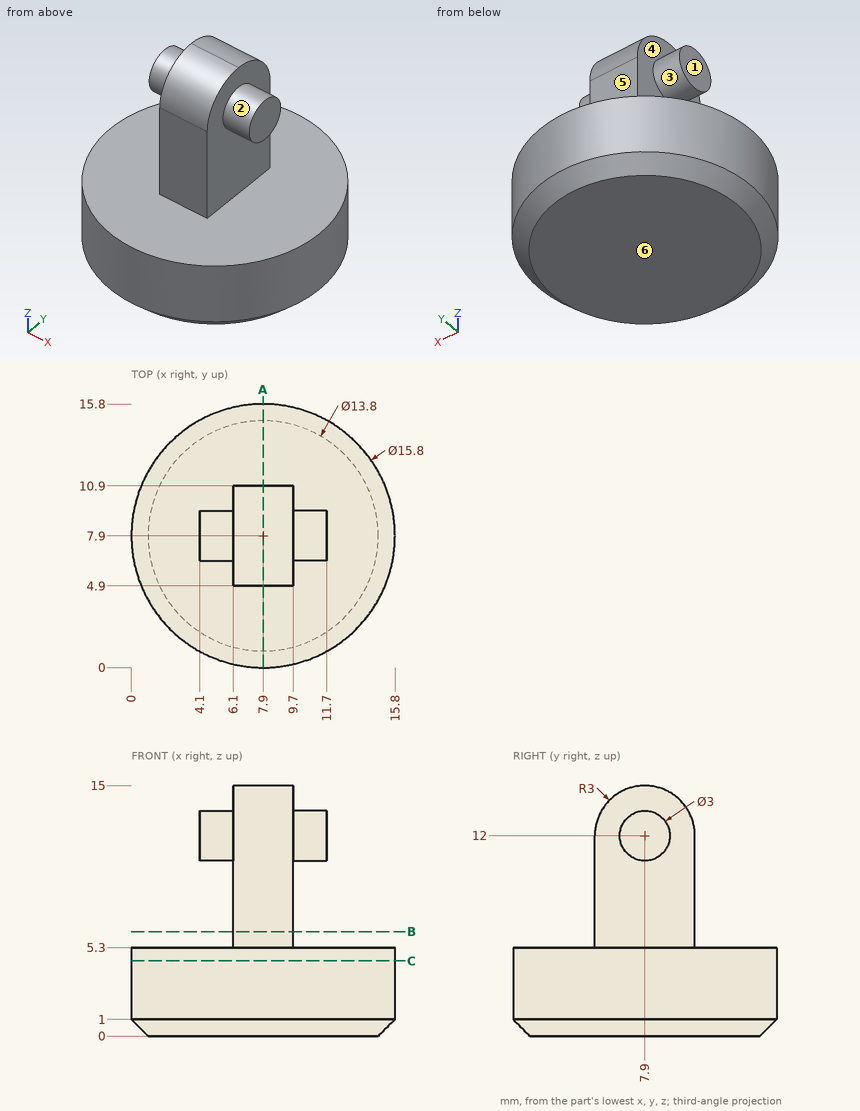
Drawing for the job (mm, zero at the part's lowest x, y, z). A direction names the side the tool comes from. Give positions to 0.01 mm unless a question says otherwise; leave off trailing zeros. Write each loop counter-clockwise with the first axis right and the second up, starting at its lowest first coordinate (ties: lowest second). Pieces come first, ordered by that corner, then holes. Notation, with made-up numbers: M 58,31 L 64,31 A18 ccw 64,57 Z; hole C 89.5,-39 d2. An arc over 180 degrees is marked long. Return JSON: item names as keys, results as strings. Group by question number.
(1) Band-saw the part on C-C (z = 4.5). Give the cut face in (x, y).
(2) Band-saw the part on B-B (z = 6.25). Give the cut face in (x, y).
(3) Mould opens along Z. For the marked faces 4, 5 and 6 say: pulls with the +Z half, pulls with the -Z half, needs draft (parallel to the pull), parting line crosses it, or undercut.
(4) Drill centre lines: L1, parallel to X at y = 5.5, z = 11.5; L2, parallel to Z at x = 5.25, y = 14; L3, parallel to Z at x = 11, y = 8. Where is each one in solid material? Low to high. Write a range as [from, to].
(5) Flat gauge pins, fed straight in: pin 1 Ø1.1 at (x, z) = (7.5, 9) entering from -Y; pin 2 Ø0.9 at (y, z) = (8.5, 12.5) entering from +X; pin 3 Ø4 at (x, y) = (4, 14) entering from -Z; pin 4 Ø1 at (y, z) = (9, 2) entering from +X. Where does each tip first touch, or does it go through?
(6) Band-saw the part on A-A (x = 7.9). Give the cut face in (y, z).
(7) 3-axis set-ups, long thin cutter, end or side, ignore diameter. For the marked faces 1, 2 and 3: which of +Z, -Z, +X, -X, +Y, -Y reach the whole face in a straight line?
Entries:
{
 "1": {"outline": "C 7.9,7.9 d15.8"},
 "2": {"outline": "M 6.1,4.9 L 9.7,4.9 L 9.7,10.9 L 6.1,10.9 Z"},
 "3": {"face 4": "undercut", "face 5": "needs draft", "face 6": "pulls with the -Z half"},
 "4": {"L1": "x = [6.1, 9.7]", "L2": "z = [0, 5.3]", "L3": "z = [0, 5.3], [10.5, 13.5]"},
 "5": {"pin 1": "stops at y = 4.9", "pin 2": "stops at x = 11.7", "pin 3": "stops at z = 0", "pin 4": "stops at x = 15.78"},
 "6": {"outline": "M 0,1 L 1,0 L 14.8,0 L 15.8,1 L 15.8,5.3 L 10.9,5.3 L 10.9,12 A3 ccw 4.9,12 L 4.9,5.3 L 0,5.3 Z"},
 "7": {"face 1": "+Z, -X, +Y, -Y", "face 2": "+X", "face 3": "-X"}
}
